The listing builds one solid part. Answer for the finished solid, in the listing's coordinates (mm). Face numbers are marked on the shaded views. Coordinates: 2 decimals unless noted, no trailing zeros. Order: outer loops, then holes, each group sorted by start corner. A loop starts at its lowest first (then second) coordinate and runs counter-clockwise, first axis right, second up. Notation, with made-up numbers: (30, 89.25) - (49, 89.25) arc R27 cw to (49, 107.25) - close; hole circle Ø11 at (42.25, 58.25). An arc over 180 degrees is marked (long way). Use a Markdown table: item, result. Add a question column.
Item 1: The part is cut by section B-B, the plane x = 0. Give the vertices of the cut face in (y, z), then the cut area to 3 significant figures.
Item 2: Find the intervals of material crossed by line 1 along X through (y, z) = (-1.25, 44.5); line 2 along X through (y, z) = (3, 8); line 3 along Z through (x, y) = (-5.5, 2.5), in increasing order.
Item 3: The part is cut by section C-C, the plane z = 8. Give the vertices of the cut face in (x, y).
Item 4: The part is cut by section D-D, the plane y = -5.25. Give the vertices of the cut face in (x, z).
Item 5: The part is cut by section A-A, the plane z = 29. Give the vertices of the cut face in (x, y).
Item 6: The mould has two halves that part along X. Classify the marked faces 1, 2 and 3: released by +X, released by -X, zero draft, split by the parting line, or undercut.
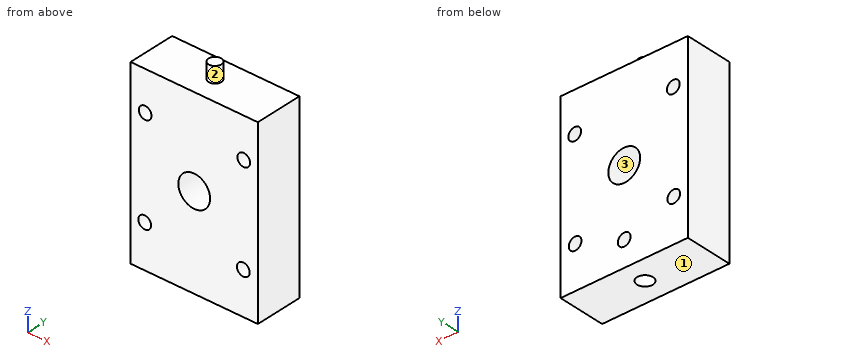
from build123d import *

# Parameters (mm, degrees)
SKETCH1_W           = 40
SKETCH1_H           = 15
BOSS_EXTRUDE1_DEPTH = 57
SKETCH2_R           = 2
BOSS_EXTRUDE2_DEPTH = 5
SKETCH3_R           = 2.5
CUT_EXTRUDE1_DEPTH  = 23
SKETCH5_R           = 2
CUT_EXTRUDE3_DEPTH  = 8
SKETCH7_R           = 5
CUT_EXTRUDE5_DEPTH  = 67.850579676
SKETCH8_R           = 2
CUT_EXTRUDE6_DEPTH  = 29


with BuildPart() as part:
    # Sketch1 → Boss-Extrude1 (new body)
    with BuildSketch(Plane.XY):
        Rectangle(SKETCH1_W, SKETCH1_H)
    extrude(amount=BOSS_EXTRUDE1_DEPTH)

    # Sketch2 → Boss-Extrude2 (add)
    with BuildSketch(Plane.XY.offset(57)):
        with Locations(Location((0, 0, 0), (0, 0, 180))):
            Circle(SKETCH2_R)
    extrude(amount=BOSS_EXTRUDE2_DEPTH)

    # Sketch3 → Cut-Extrude1 (cut)
    with BuildSketch(Plane(origin=(0, 0, 0), x_dir=(-1, 0, 0), z_dir=(0, 0, -1))):
        Circle(SKETCH3_R)
    extrude(amount=-CUT_EXTRUDE1_DEPTH, mode=Mode.SUBTRACT)

    # Sketch5 → Cut-Extrude3 (cut)
    with BuildSketch(Plane(origin=(0, 7.5, 0), x_dir=(1, 0, 0), z_dir=(0, 1, 0))):
        with Locations(Location((0, -8, 0), (0, 0, 270))):
            Circle(SKETCH5_R)
    extrude(amount=-CUT_EXTRUDE3_DEPTH, mode=Mode.SUBTRACT)

    # Sketch7 → Cut-Extrude5 (cut, through all)
    with BuildSketch(Plane(origin=(0, -7.5, 0), x_dir=(-1, 0, 0), z_dir=(0, -1, 0))):
        with Locations(Location((0, -29, 0), (0, 0, 90))):
            Circle(SKETCH7_R)
    extrude(amount=-CUT_EXTRUDE5_DEPTH, mode=Mode.SUBTRACT)

    # Sketch8 → Cut-Extrude6 (cut)
    with BuildSketch(Plane(origin=(0, -7.5, 0), x_dir=(-1, 0, 0), z_dir=(0, -1, 0))):
        with Locations(Location((-15.433459582, -13.433744017, 0), (0, 0, 90))):
            Circle(SKETCH8_R)
        with Locations(Location((-15.566255983, -44.433459582, 0), (0, 0, 90))):
            Circle(SKETCH8_R)
        with Locations(Location((15.433459582, -44.566255983, 0), (0, 0, 90))):
            Circle(SKETCH8_R)
        with Locations(Location((15.566255983, -13.566540418, 0), (0, 0, 90))):
            Circle(SKETCH8_R)
    extrude(amount=-CUT_EXTRUDE6_DEPTH, mode=Mode.SUBTRACT)


solid = part.part
Solution:
| question | item | result |
|---|---|---|
| 1 | outline | (-7.5, 0) - (-2.5, 0) - (-2.5, 23) - (2.5, 23) - (2.5, 10) - (7.5, 10) - (7.5, 24) - (-7.5, 24) - close; (-7.5, 34) - (7.5, 34) - (7.5, 57) - (2, 57) - (2, 62) - (-2, 62) - (-2, 57) - (-7.5, 57) - close; (2.5, 0) - (7.5, 0) - (7.5, 6) - (2.5, 6) - close |
| 1 | area | 590 mm2 |
| 2 | line 1 | x = -20 to -17.43, -13.43 to 13.57, 17.57 to 20 |
| 2 | line 2 | x = -20 to -2, 2 to 20 |
| 2 | line 3 | z = 0 to 57 |
| 3 | outline | (-20, -7.5) - (20, -7.5) - (20, 7.5) - (2, 7.5) - (2, 1.5) arc R2.5 cw (long way) to (-2, 1.5) - (-2, 7.5) - (-20, 7.5) - close |
| 4 | outline | (-20, 0) - (20, 0) - (20, 57) - (-20, 57) - close; hole circle Ø4 at (-15.57, 13.57); hole circle Ø4 at (-15.43, 44.57); hole circle Ø10 at (0, 29); hole circle Ø4 at (15.43, 13.43); hole circle Ø4 at (15.57, 44.43) |
| 5 | outline | (-20, -7.5) - (-5, -7.5) - (-5, 7.5) - (-20, 7.5) - close; (5, -7.5) - (20, -7.5) - (20, 7.5) - (5, 7.5) - close |
| 6 | face 1 | zero draft |
| 6 | face 2 | split by the parting line |
| 6 | face 3 | undercut |
